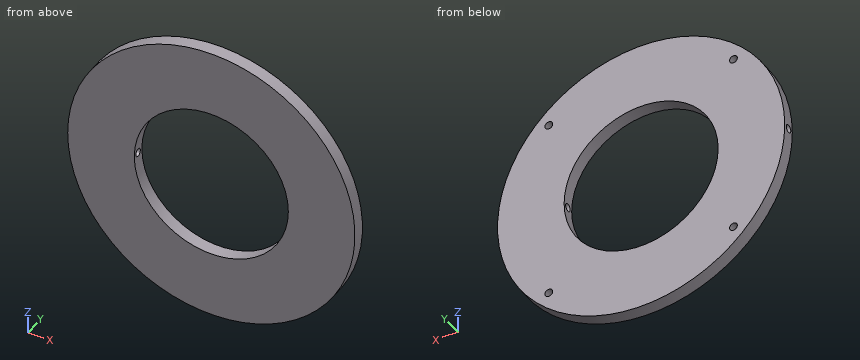
Autodesk Inventor part; units mm, degrees
ref_plane "Work Plane1" through (50, 0, 0) normal (1, 0, 0) x (0, 1, 0)
ref_plane "XZ Plane" through (0, 0, 0) normal (0, 1, 0) x (-1, 0, 0)
ref_plane "XY Plane" through (0, 0, 0) normal (0, 0, 1) x (1, 0, 0)
sketch "Sketch1" plane through (0, 0, 0) normal (0, 1, 0) x (-1, 0, 0)
  circle A0 centre (0, 0) radius 55
  circle A1 centre (0, 0) radius 29.5
  dimension "d0" = 110
  dimension "d1" = 59
extrude "Extrusion1" add sketch "Sketch1" along normal blind 5
ref_plane "Work Plane1" through (50, 0, 0) normal (1, 0, 0) x (0, 1, 0)
sketch "Sketch2" plane through (50, 0, 0) normal (1, 0, 0) x (0, 1, 0)
  circle A0 centre (2.5, 0) radius 1.5
  line L0 (5, -55) -> (5, 55)
  point P0 (0, 0)
  dimension "d5" = 3
  dimension "d6" = 2.5
hole "Hole1" at (50, 2.5, 0) direction (-1, 0, 0) diameter 3 end through all
sketch "Sketch6" plane through (0, 5, 0) normal (0, 1, 0) x (1, 0, 0)
  circle A0 centre (-35.3554, 35.3553) radius 1.5
  circle A1 centre (35.3553, 35.3554) radius 1.5
  circle A2 centre (35.3554, -35.3553) radius 1.5
  circle A3 centre (-35.3553, -35.3554) radius 1.5
  point P0 (0, 0)
  dimension "d30" = 3
  dimension "d31" = 50
  dimension "d32" = 3
  dimension "d33" = 50
  dimension "d34" = 90
  dimension "d35" = 35.3553
  dimension "d36" = 3
  dimension "d37" = 3
  dimension "d38" = 50
  dimension "d39" = 90
  dimension "d40" = 50
  dimension "d41" = 90
extrude "Extrusion6" cut sketch "Sketch6" against normal blind 3
properties part number "Mirror Support 2"
Geometry: final body of the model. Coordinates: model frame, mm. Give positions to 0.01 mm unless a question says otherwise; leave off trailing zeros. Order: outer loops, then holes, each group sorted by start corner. A loop starts at its lowest first (then second) coordinate and runs counter-clockwise, first axis right, second up. Notation, with made-up numbers: M 50,11 L 98,11 A16 ccw 98,34 Z; hole C 37.25,-26 d5. An arc over 180 degrees is marked long. Answer as CSV lines item,"result". Start each with the question number.
1) Line query: line 1 (Z direction, x = -35, y = 2.8); line 2 (Z direction, x = 0, y = 1.7); line 3 (X direction, y = 3.05, z = -1). Output: solid intervals per line, ascending. Write a range as from..to.
2) Cut plane C-C (z = -20). Output: boundary loops of the cut face in (x, y).
3) Cut plane A-A (z = 0). Output: boundary loops of the cut face in (x, y), then the cut area to 3 significant figures.
4) Cut plane B-B (x = 0). Output: boundary loops of the cut face in (y, z), then the cut area to 3 significant figures.
5) First-contact query: P1, Ø2.5, axis at x = 35.36, z = 35.36, coming from the +Y side; P2, Ø1.5, axis at y = 2, z = -0.5, coming from the -X side; P3, Ø3, axis at y = 2.5, z = 13.5, coming from the -X side. Flat tips, straight axial feed; report the tip coordinate or a pass-through.
6) Cut plane D-D (x = -40). Output: boundary loops of the cut face in (y, z).
Findings below:
1,line 1,"z = -42.43..-36.81, -33.9..-1.47, 1.47..33.9, 36.81..42.43"
1,line 2,"z = -55..-29.5, 29.5..55"
1,line 3,"x = 50..54.99"
2,outline,"M -51.23,0 L -21.69,0 L -21.69,5 L -51.23,5 Z; M 21.69,0 L 51.23,0 L 51.23,5 L 21.69,5 Z"
3,outline,"M -55,0 L -29.5,0 L -29.5,1 L -55,1 Z; M -55,4 L -29.5,4 L -29.5,5 L -55,5 Z; M 29.5,0 L 55,0 L 55,5 L 29.5,5 L 29.5,4 L 50,4 L 50,1 L 29.5,1 Z"
3,area,"117 mm²"
4,outline,"M 0,-55 L 5,-55 L 5,-29.5 L 0,-29.5 Z; M 0,29.5 L 5,29.5 L 5,55 L 0,55 Z"
4,area,"255 mm²"
5,P1,"stops at y = 2"
5,P2,"stops at x = 50"
5,P3,"stops at x = -53.67"
6,outline,"M 0,-37.75 L 5,-37.75 L 5,37.75 L 0,37.75 Z; hole C 2.5,0 d3"
